Read the model definition and answer for the solid it produces. Units are mm, in the model's axes. Face numbers are marked on the shaded views. A direction names the side the tool comes from. Coordinates: 2 decimals unless noted, no trailing zeros. Order: outer loops, then holes, each group sorted by start corner. A loop starts at its lowest first (then second) coordinate and runs counter-clockwise, first axis right, second up. Notation, with made-up numbers: (78.5, 28) - (118.5, 28) arc R17 cw to (118.5, 60) - close; hole circle Ø5 at (46, 65.5). An arc over 180 degrees is marked (long way). Write item = value, one per line.
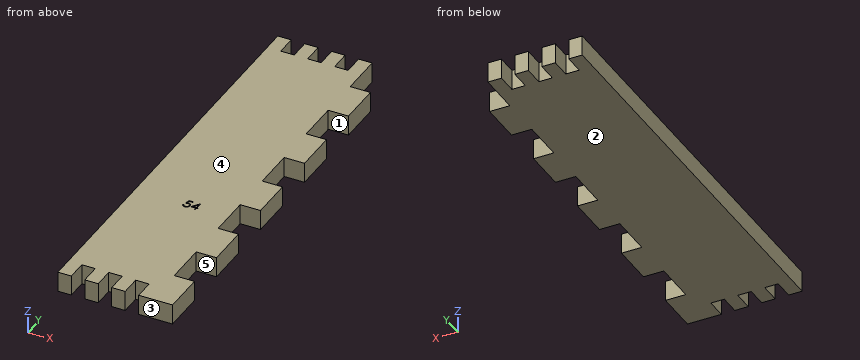
from build123d import *

# Parameters (mm, degrees)
BOSS_EXTRUDE7_DEPTH = 6.2
CUT_EXTRUDE10_DEPTH = 1


with BuildPart() as part:
    # Sketch1 → Boss-Extrude7 (new body)
    with BuildSketch(Plane.XY):
        Polygon((4.11, 130), (0, 130), (0, 0), (4.11, 0), (4.11, 6.2), (8.22, 6.2), (8.22, 0), (12.33, 0), (12.33, 6.2), (16.44, 6.2), (16.44, 0), (20.55, 0), (20.55, 6.2), (24.66, 6.2), (24.66, 0), (35, 0), (35, 13), (28.8, 13), (28.8, 26), (35, 26), (35, 39), (28.8, 39), (28.8, 52), (35, 52), (35, 65), (28.8, 65), (28.8, 78), (35, 78), (35, 91), (28.8, 91), (28.8, 104), (35, 104), (35, 117), (28.8, 117), (28.8, 130), (24.66, 130), (24.66, 123.8), (20.55, 123.8), (20.55, 130), (16.44, 130), (16.44, 123.8), (12.33, 123.8), (12.33, 130), (8.22, 130), (8.22, 123.8), (4.11, 123.8), align=None)
    extrude(amount=BOSS_EXTRUDE7_DEPTH)

    # Sketch7 → Cut-Extrude10 (cut)
    with BuildSketch(Plane.XY.offset(6.2)):
        with BuildLine():
            Line((16.852728424, 47.419269681), (16.852728424, 47.093628655))
            Line((16.852728424, 47.093628655), (15.772770491, 47.093628655))
            Line((15.772770491, 47.093628655), (15.601681749, 46.25853751))
            add(Edge.make_bspline(
                [(15.601681749, 46.25853751), (15.635296721, 46.267817828), (15.700420412, 46.285796976), (15.796541143, 46.305759353), (15.887792642, 46.317793006), (15.947006728, 46.319436124), (15.975660115, 46.32023122)],
                knots=[0, 0, 0, 0, 0.000104595, 0.000202637, 0.000294305, 0.000380252, 0.000380252, 0.000380252, 0.000380252], degree=3))
            add(Edge.make_bspline(
                [(15.975660115, 46.32023122), (16.01111465, 46.319463835), (16.080827125, 46.317954965), (16.182825312, 46.303466216), (16.28019158, 46.280660722), (16.372722301, 46.248801392), (16.460588658, 46.208061848), (16.542982232, 46.157171188), (16.621139767, 46.097723095), (16.69365912, 46.029374405), (16.759449028, 45.954152653), (16.81729389, 45.873273727), (16.866427097, 45.787523633), (16.905942925, 45.696083081), (16.937497285, 45.599962992), (16.958499452, 45.498152006), (16.972484609, 45.391609783), (16.97404706, 45.318762066), (16.974843809, 45.281614433)],
                knots=[0, 0, 0, 0, 0.000106308, 0.000209029, 0.000308378, 0.000405929, 0.000502102, 0.000598312, 0.00069588, 0.000796219, 0.000896736, 0.000995218, 0.001094066, 0.001192613, 0.001293582, 0.001396995, 0.001504047, 0.001615439, 0.001615439, 0.001615439, 0.001615439], degree=3))
            add(Edge.make_bspline(
                [(16.974843809, 45.281614433), (16.97424049, 45.255740704), (16.973042007, 45.204342908), (16.966947288, 45.128012098), (16.955212746, 45.053297242), (16.939457739, 44.980188429), (16.919008546, 44.90882407), (16.894253475, 44.838999899), (16.863958507, 44.771150505), (16.830728617, 44.704633897), (16.793312169, 44.640953823), (16.751784523, 44.581400813), (16.707910113, 44.525081501), (16.660701142, 44.4725999), (16.609718811, 44.424300877), (16.555580555, 44.379897793), (16.498718374, 44.338639729), (16.438252547, 44.302201438), (16.375530438, 44.268670756), (16.309646269, 44.241162976), (16.242099777, 44.216569854), (16.171918783, 44.196966925), (16.099262253, 44.181606679), (16.024010421, 44.171173992), (15.946557956, 44.163575366), (15.894057051, 44.1630997), (15.867537118, 44.162859425)],
                knots=[0, 0, 0, 0, 7.7636e-05, 0.000154223, 0.000229512, 0.000304362, 0.000378447, 0.000452077, 0.000526407, 0.000601214, 0.00067506, 0.000747747, 0.00081887, 0.000889121, 0.000959302, 0.001029336, 0.001099058, 0.00116985, 0.001240974, 0.00131221, 0.00138383, 0.001456517, 0.001530612, 0.001606437, 0.001684346, 0.001763871, 0.001763871, 0.001763871, 0.001763871], degree=3))
            add(Edge.make_bspline(
                [(15.867537118, 44.162859425), (15.835901254, 44.163486113), (15.773661429, 44.164719049), (15.682474915, 44.177617247), (15.594740951, 44.196090228), (15.511165788, 44.223881701), (15.431000427, 44.258704462), (15.355324104, 44.30271556), (15.28220315, 44.352589461), (15.214610088, 44.41144521), (15.151875614, 44.475775865), (15.095717567, 44.545587439), (15.045703536, 44.619727719), (15.002634437, 44.698556758), (14.965896947, 44.781867426), (14.937036207, 44.869971862), (14.913742271, 44.962409723), (14.903887597, 45.026048979), (14.89888227, 45.058372245)],
                knots=[0, 0, 0, 0, 9.4843e-05, 0.000186593, 0.000275792, 0.000363484, 0.000450342, 0.000537514, 0.000625728, 0.000715478, 0.000805885, 0.000894984, 0.00098389, 0.001073836, 0.001164117, 0.001256635, 0.001351658, 0.001449737, 0.001449737, 0.001449737, 0.001449737], degree=3))
            Line((14.89888227, 45.058372245), (15.183818168, 45.058372245))
            add(Edge.make_bspline(
                [(15.183818168, 45.058372245), (15.190829073, 45.028095035), (15.204304423, 44.969900555), (15.233882495, 44.888138553), (15.270046539, 44.815277543), (15.313049055, 44.750353706), (15.364348012, 44.69373983), (15.422885422, 44.64328721), (15.488515143, 44.5977712), (15.561443286, 44.559831975), (15.638380866, 44.52747532), (15.718905406, 44.50592914), (15.800824349, 44.490779044), (15.856231156, 44.489262518), (15.884073576, 44.48850045)],
                knots=[0, 0, 0, 0, 9.3172e-05, 0.000179081, 0.000260145, 0.000336703, 0.000411917, 0.000488562, 0.000568128, 0.000650923, 0.00073478, 0.000817953, 0.000900557, 0.000983994, 0.000983994, 0.000983994, 0.000983994], degree=3))
            add(Edge.make_bspline(
                [(15.884073576, 44.48850045), (15.911250165, 44.489245013), (15.964761091, 44.490711063), (16.04351142, 44.501995024), (16.11954167, 44.519373678), (16.19210163, 44.545381332), (16.262461026, 44.57699047), (16.32884009, 44.617553432), (16.393159128, 44.66423502), (16.453418935, 44.717717106), (16.508609007, 44.7766539), (16.557373488, 44.839679821), (16.597992545, 44.906914389), (16.632222773, 44.977193606), (16.658215408, 45.051287726), (16.676758298, 45.128849506), (16.687646787, 45.210070524), (16.689144643, 45.265469112), (16.689907911, 45.293698768)],
                knots=[0, 0, 0, 0, 8.15e-05, 0.000160473, 0.000238226, 0.000315066, 0.000391338, 0.000469218, 0.000547964, 0.000629516, 0.000710512, 0.000789892, 0.000868102, 0.000945761, 0.001024012, 0.00110315, 0.001184644, 0.001269321, 0.001269321, 0.001269321, 0.001269321], degree=3))
            add(Edge.make_bspline(
                [(16.689907911, 45.293698768), (16.689310576, 45.319167485), (16.688141378, 45.369018876), (16.678588646, 45.441952442), (16.661972536, 45.510961559), (16.638909445, 45.576379471), (16.60962732, 45.638267879), (16.573843879, 45.696690655), (16.530887583, 45.750877776), (16.481818512, 45.800854592), (16.428063004, 45.846978157), (16.36869618, 45.886297436), (16.304960389, 45.919375418), (16.237623538, 45.947921388), (16.165083952, 45.968423493), (16.08877815, 45.983815789), (16.007882136, 45.992719725), (15.952573012, 45.993955152), (15.924142687, 45.994590194)],
                knots=[0, 0, 0, 0, 7.6388e-05, 0.000149519, 0.000220172, 0.000288967, 0.000357247, 0.000425206, 0.000494043, 0.000564207, 0.000635056, 0.000706145, 0.000777268, 0.000850264, 0.000925136, 0.001002969, 0.001083601, 0.001168886, 0.001168886, 0.001168886, 0.001168886], degree=3))
            add(Edge.make_bspline(
                [(15.924142687, 45.994590194), (15.899532873, 45.994063515), (15.84871985, 45.992976056), (15.770775572, 45.984969162), (15.68886808, 45.972052088), (15.603311359, 45.954284564), (15.51384847, 45.931033516), (15.420668206, 45.903171076), (15.32357465, 45.869858977), (15.258153572, 45.844701897), (15.224523296, 45.831769681)],
                knots=[0, 0, 0, 0, 7.3822e-05, 0.000152423, 0.000234822, 0.000322511, 0.00041445, 0.000512043, 0.000614219, 0.000722306, 0.000722306, 0.000722306, 0.000722306], degree=3))
            Line((15.224523296, 45.831769681), (15.550164321, 47.419269681))
            Line((15.550164321, 47.419269681), (16.852728424, 47.419269681))
        make_face()
        Polygon((19.033632871, 47.500679937), (19.091510475, 47.500679937), (19.091510475, 45.302603014), (19.457856629, 45.302603014), (19.457856629, 44.976961989), (19.091510475, 44.976961989), (19.091510475, 44.244269681), (18.806574578, 44.244269681), (18.806574578, 44.976961989), (17.300484834, 44.976961989), align=None)
        Polygon((18.806574578, 45.302603014), (18.806574578, 46.681489232), (17.860180347, 45.302603014), align=None, mode=Mode.SUBTRACT)
    extrude(amount=-CUT_EXTRUDE10_DEPTH, mode=Mode.SUBTRACT)


solid = part.part
1) For the marked faces 4 and 5, determine the directions among +Z, -Z, +X, -X, +Y, -Y from which every point of the face is accessible in a straight line to the end or side of a thin tool.
Returned:
face_4 = +Z, +X, -X, +Y, -Y
face_5 = +Z, -Z, +X
2) Straight lines are drawn through the part: line 1 along Y through (x, z) = (32, 0.5); line 2 along X through (y, z) = (21.5, 0.75); line 3 along Y through (x, z) = (22.5, 3). For each, find the intervals that lie inside material, in ascending order. Write a range as from..to.
Returned:
line_1 = 0..13, 26..39, 52..65, 78..91, 104..117
line_2 = 0..28.8
line_3 = 6.2..123.8
3) The part is cut by section B-B (y = 76.5). Determine the outline of the cut face in (x, z).
Returned:
outline = (0, 0) - (28.8, 0) - (28.8, 6.2) - (0, 6.2) - close
4) Flat-ended cylindrical pins translate along their axes: pin 1 Ø1.9 at (x, z) = (33, 3.5) entering from +Y; pin 2 Ø0.8 at (y, z) = (46, 5.5) entering from +X. Find the tip coordinate at first contact, or state that the pin passes through.
Returned:
pin_1 = 117
pin_2 = 28.8
5) The part is cut by section A-A (x = 13.5). Determine the outline of the cut face in (y, z), and give its area (3 significant figures).
Returned:
outline = (6.2, 0) - (123.8, 0) - (123.8, 6.2) - (6.2, 6.2) - close
area = 729 mm^2
6) Determine the mould class of the marked faces 1, 2 and 3 for opening direction Y: pulls with the +Y half, pulls with the -Y half, needs draft (parallel to the pull), parting line crosses it, or undercut.
Returned:
face_1 = undercut
face_2 = needs draft
face_3 = pulls with the -Y half
